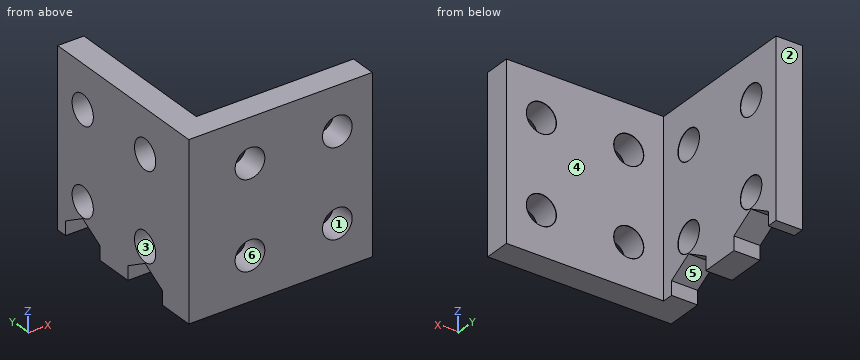
from build123d import *

# Parameters (mm, degrees)
BOSS_EXTRUDE1_DEPTH            = 20
M3_CLEARANCE_HOLE1_D           = 3.4
M3_CLEARANCE_HOLE1_CSINK_D     = 3.45
M3_CLEARANCE_HOLE1_CSINK_ANGLE = 90
M3_CLEARANCE_HOLE2_D           = 3.4
M3_CLEARANCE_HOLE2_CSINK_D     = 3.45
M3_CLEARANCE_HOLE2_CSINK_ANGLE = 90
CUT_EXTRUDE1_DEPTH             = 3


with BuildPart() as part:
    # Sketch1 → Boss-Extrude1 (new body)
    with BuildSketch(Plane.XY):
        Polygon((0, 21), (0, 0), (21, 0), (21, 3), (3, 3), (3, 21), align=None)
    extrude(amount=BOSS_EXTRUDE1_DEPTH)

    # M3 Clearance Hole1 (through all)
    with Locations(Plane(origin=(0, 3, 0), x_dir=(1, 0, 0), z_dir=(0, 1, 0))):
        with Locations((7, -15), (7, -5), (17, -5), (17, -15)):
            CounterSinkHole(M3_CLEARANCE_HOLE1_D / 2, M3_CLEARANCE_HOLE1_CSINK_D / 2, counter_sink_angle=M3_CLEARANCE_HOLE1_CSINK_ANGLE)

    # M3 Clearance Hole2 (through all)
    with Locations(Plane(origin=(3, 0, 0), x_dir=(0, 0, -1), z_dir=(1, 0, 0))):
        with Locations((-15, 7), (-5, 7), (-5, 17), (-15, 17)):
            CounterSinkHole(M3_CLEARANCE_HOLE2_D / 2, M3_CLEARANCE_HOLE2_CSINK_D / 2, counter_sink_angle=M3_CLEARANCE_HOLE2_CSINK_ANGLE)

    # Sketch6 → Cut-Extrude1 (cut)
    with BuildSketch(Plane(origin=(3, 0, 0), x_dir=(0, 0, -1), z_dir=(1, 0, 0))):
        Polygon((0, 9.75), (-1.58771324, 9.75), (-3.175426481, 7), (-1.58771324, 4.25), (0, 4.25), align=None)
        Polygon((-1.58771324, 14.25), (0, 14.25), (0, 19.75), (-1.58771324, 19.75), (-3.175426481, 17), align=None)
    extrude(amount=-CUT_EXTRUDE1_DEPTH, mode=Mode.SUBTRACT)


solid = part.part
Here's how the part is built. I have some questions about the finished solid (model axes, mm). Face numbers are marked on the shaded views. A direction names the side the tool comes from. Round coordinates to 2 decimals unless told otherwise and drop trailing zeros. Write each loop counter-clockwise with the first axis right and the second up, starting at its lowest first coordinate (ties: lowest second). Pieces come first, ordered by that corner, then holes.
1. Suppose I cut it at C-C (z = 15). State how many separate pieces and enclosed holes the cut face has, and give its area (3 significant figures).
2. Suppose I cut it at B-B (y = 2.25). List the corners of the cut face in (x, z) for me, and give its area (3 significant figures).
3. Will these pins go through, and if not, where does the flat tip stop? pin 1 Ø10 at (x, z) = (10.5, 9.5) entering from +Y; pin 2 Ø2 at (y, z) = (18.5, 16.5) entering from +X.
4. I need wall thicknesses on L1, parallel to Z at x = 7, y = 1.4; L2, parallel to Y at x = 0.8, z = 15. Which ranges of each line are inside material? Lowest first, please.
5. Suppose I cut it at A-A (x = 17). List the corners of the cut face in (y, z) for me (3 decimals), and give its area (3 significant figures).
6. If we mould it in two halves opening along Y, with no side actions, what happens to the marked faces 1, 2 and 3? For each: released by +Y, released by -Y, zero draft, split by the parting line, or undercut.
7. For the marked faces 4, 5 and 6, which set-ups out of +Z, -Z, +X, -X, +Y, -Y let a thin tool reach every point of the face, with its end or its side?
Answer sheet:
1. separate pieces: 5
1. enclosed holes: 0
1. area: 76.2 mm2
2. outline: (0, 0) - (21, 0) - (21, 20) - (0, 20) - close; hole circle Ø3.4 at (7, 5); hole circle Ø3.4 at (7, 15); hole circle Ø3.4 at (17, 5); hole circle Ø3.4 at (17, 15)
2. area: 384 mm2
3. pin 1: stops at y = 3
3. pin 2: stops at x = 3
4. L1: z = 0 to 3.3, 6.7 to 13.3, 16.7 to 20
4. L2: y = 0 to 5.3, 8.7 to 15.3, 18.7 to 21
5. outline: (0, 0) - (3, 0) - (3, 3.275) - (2.975, 3.3) - (0, 3.3) - close; (0, 6.7) - (2.975, 6.7) - (3, 6.725) - (3, 13.275) - (2.975, 13.3) - (0, 13.3) - close; (0, 16.7) - (2.975, 16.7) - (3, 16.725) - (3, 20) - (0, 20) - close
5. area: 39.6 mm2
6. face 1: zero draft
6. face 2: released by +Y
6. face 3: undercut
7. face 4: +Z, -Z, +X, +Y
7. face 5: -Z, +X, -X
7. face 6: +Y, -Y
